Could you check a few things on this drawing? It's one solid part, dimensions in mm from its lowest x, y, z. Coordinates: 2 decimals unless noted, no trailing zeros. Write each loop counter-clockwise with the first axis right and the second up, starting at its lowest first coordinate (ties: lowest second). Pieces come first, ordered by that corner, then holes.
Item 1: I'm going to push flat-ended pins straight in: P1, Ø1.3, axis at x = 376.5, y = 3, coming from the -Z side; P2, Ø1.5, axis at x = 132, y = 2, coming from the -Z side; P3, Ø1.3, axis at y = 1.5, z = 6, coming from the +X side; P4, Ø1.3, axis at y = 3, z = 5.5, coming from the -X side. Where does each tip first touch, or does it pass through?
Item 2: Please list where these lines run through material, in increasing order: line 1 (X direction, y = 2.75, z = 43.1); line 2 (X direction, y = 1, z = 23); line 3 (X direction, y = 3.35, z = 214.5).
Item 3: I want a section at B-B (y = 3.3). Count the separate pieces of the cut face and the enclosed holes in it, and give its area (3 significant figures).
Item 4: I want a section at A-A (z = 76). Please give me the cut outline in (x, y).
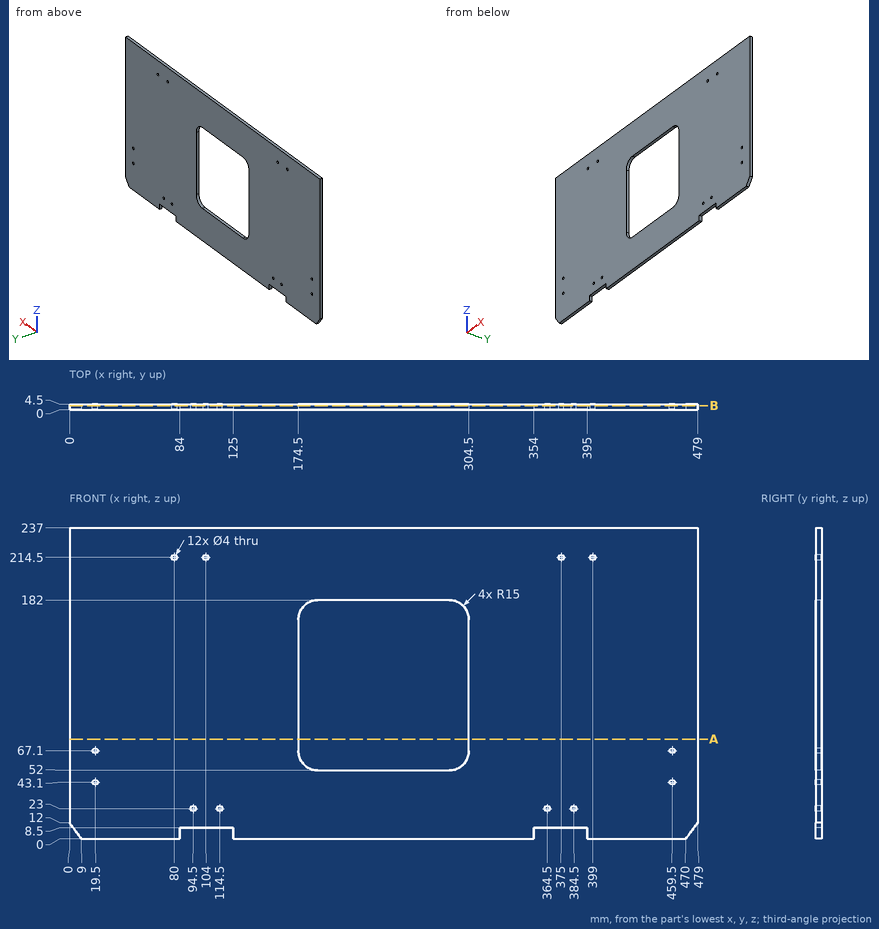
Answer:
1. P1: stops at z = 8.5
1. P2: stops at z = 0
1. P3: stops at x = 474.99
1. P4: stops at x = 4.39
2. line 1: x = 0 to 17.5, 21.5 to 457.5, 461.5 to 479
2. line 2: x = 0 to 92.5, 96.5 to 112.5, 116.5 to 362.5, 366.5 to 382.5, 386.5 to 479
2. line 3: x = 0 to 78, 82 to 102, 106 to 373, 377 to 397, 401 to 479
3. separate pieces: 1
3. enclosed holes: 13
3. area: 95,900 mm2
4. outline: (0, 0) - (174.5, 0) - (174.5, 4.5) - (0, 4.5) - close; (304.5, 0) - (479, 0) - (479, 4.5) - (304.5, 4.5) - close
